```python
from build123d import *
from OCP.BRepFilletAPI import BRepFilletAPI_MakeChamfer

# Parameters (mm, degrees)
SKETCH1_W                      = 70
SKETCH1_H                      = 70
BOSS_EXTRUDE1_DEPTH            = 10
M3_CLEARANCE_HOLE1_D           = 3.4
M3_CLEARANCE_HOLE1_CSINK_D     = 3.65
M3_CLEARANCE_HOLE1_CSINK_ANGLE = 90
SKETCH14_W                     = 70
SKETCH14_H                     = 10
BOSS_EXTRUDE2_DEPTH            = 63
SKETCH13_W                     = 186
SKETCH13_H                     = 106
BOSS_EXTRUDE3_DEPTH            = 10
CHAMFER1_SIZE                  = 40
CHAMFER1_SIZE2                 = 53
HOLE1_D                        = 4.5
HOLE1_DEPTH                    = 9
HOLE1_CBORE_D                  = 5.2
HOLE1_CBORE_DEPTH              = 2
CHAMFER2_SIZE                  = 2
CHAMFER2_SIZE_2                = 0.35


with BuildPart() as part:
    # Sketch1 → Boss-Extrude1 (new body)
    with BuildSketch(Plane.XY):
        Rectangle(SKETCH1_W, SKETCH1_H)
    extrude(amount=BOSS_EXTRUDE1_DEPTH)

    # M3 Clearance Hole1 (through all)
    with Locations(Plane.XY.offset(10)):
        with Locations((6.314276634, -15.244012286), (10.044563579, 13.090330115), (-16.358840213, 2.153682172)):
            CounterSinkHole(M3_CLEARANCE_HOLE1_D / 2, M3_CLEARANCE_HOLE1_CSINK_D / 2, counter_sink_angle=M3_CLEARANCE_HOLE1_CSINK_ANGLE)

    # Sketch14 → Boss-Extrude2 (add)
    with BuildSketch(Plane.XZ.offset(35)):
        with Locations((0, 5)):
            Rectangle(SKETCH14_W, SKETCH14_H)
    extrude(amount=BOSS_EXTRUDE2_DEPTH)

    # Sketch13 → Boss-Extrude3 (add)
    with BuildSketch(Plane.XZ.offset(98)):
        with Locations((0, -43)):
            Rectangle(SKETCH13_W, SKETCH13_H)
    extrude(amount=-BOSS_EXTRUDE3_DEPTH)

    # Chamfer1
    chamfer1_edges = [part.edges().sort_by_distance(p)[0] for p in [
        (0, -88, 0),
    ]]
    chamfer1_side = [part.faces().sort_by_distance(p)[0] for p in [
        (0, -88, -44.766933109),
    ]]
    chamfer(chamfer1_edges, length=CHAMFER1_SIZE, length2=CHAMFER1_SIZE2, reference=chamfer1_side[0])

    # Hole1
    with Locations(Plane(origin=(0, -88, 0), x_dir=(1, 0, 0), z_dir=(0, 1, 0))):
        with Locations((-89, 7.3), (-89, 82.2), (-40.8, 6), (-73.8, 58.1), (-45.9, 58.1)):
            CounterBoreHole(HOLE1_D / 2, HOLE1_CBORE_D / 2, HOLE1_CBORE_DEPTH, depth=HOLE1_DEPTH)

    # Chamfer2
    chamfer2_edges_1 = [part.edges().sort_by_distance(p)[0] for p in [
        (-43.4, -90, -6),
    ]]
    chamfer2_side_1 = [part.faces().sort_by_distance(p)[0] for p in [
        (-43.4, -89.993, -6),
    ]]
    chamfer2_edges_2 = [part.edges().sort_by_distance(p)[0] for p in [
        (-91.6, -90, -82.2),
    ]]
    chamfer2_side_2 = [part.faces().sort_by_distance(p)[0] for p in [
        (-91.6, -89.993, -82.2),
    ]]
    chamfer2_edges_3 = [part.edges().sort_by_distance(p)[0] for p in [
        (-91.6, -90, -7.3),
    ]]
    chamfer2_side_3 = [part.faces().sort_by_distance(p)[0] for p in [
        (-91.6, -89.993, -7.3),
    ]]
    chamfer2_edges_4 = [part.edges().sort_by_distance(p)[0] for p in [
        (-48.5, -90, -58.1),
    ]]
    chamfer2_side_4 = [part.faces().sort_by_distance(p)[0] for p in [
        (-48.5, -89.993, -58.1),
    ]]
    chamfer2_edges_5 = [part.edges().sort_by_distance(p)[0] for p in [
        (-76.4, -90, -58.1),
    ]]
    chamfer2_side_5 = [part.faces().sort_by_distance(p)[0] for p in [
        (-76.4, -89.993, -58.1),
    ]]
    chamfer2 = BRepFilletAPI_MakeChamfer(part.part.solid().wrapped)
    for e in chamfer2_edges_1:
        chamfer2.Add(CHAMFER2_SIZE - 0.0001, CHAMFER2_SIZE_2 - 0.0001, e.wrapped, chamfer2_side_1[0].wrapped)
    for e in chamfer2_edges_2:
        chamfer2.Add(CHAMFER2_SIZE - 0.0001, CHAMFER2_SIZE_2 - 0.0001, e.wrapped, chamfer2_side_2[0].wrapped)
    for e in chamfer2_edges_3:
        chamfer2.Add(CHAMFER2_SIZE - 0.0001, CHAMFER2_SIZE_2 - 0.0001, e.wrapped, chamfer2_side_3[0].wrapped)
    for e in chamfer2_edges_4:
        chamfer2.Add(CHAMFER2_SIZE - 0.0001, CHAMFER2_SIZE_2 - 0.0001, e.wrapped, chamfer2_side_4[0].wrapped)
    for e in chamfer2_edges_5:
        chamfer2.Add(CHAMFER2_SIZE - 0.0001, CHAMFER2_SIZE_2 - 0.0001, e.wrapped, chamfer2_side_5[0].wrapped)
    add(Compound.cast(chamfer2.Shape()), mode=Mode.REPLACE)  # a hair under: the kernel refuses the full size


solid = part.part
```
Part model, mm, in its own coordinate system. A direction names the side the tool comes from. Coordinates: 2 decimals unless noted, no trailing zeros. Write each loop counter-clockwise with the first axis right and the second up, starting at its lowest first coordinate (ties: lowest second). Pieces come first, ordered by that corner, then holes.
Item 1: Mould opens along Z. For faces 4 (the face through (0, 0, 0)), 5 (the face through (-89, -97, -82)), 6 (the face through (93, -93, -44)) say: released by +Z, released by -Z, zero draft, split by the parting line, or undercut.
Item 2: Slice it at C-C (y = -5). Write the cut outline in (x, z).
Item 3: Probe line 1 (X direction, y = -95.5, z = -58.1); line 2 (X direction, y = -93.25, z = -6); line 3 (X direction, y = -81, z = -14). List the from-to ranges inside material, lowest first.
Item 4: Slice it at A-A (x = -4.5). Write the cut outline in (y, z).
Item 5: Which spindle directions (+Z, -Z, +X, -X, +Y, -Y) get a long thin tool onto all of the face, cutting with end or side? Do faces 1 (the face through (-1, -47, 10)), 2 (the face through (-46, -97, -58)), 3 (the face through (-35, -39, 1)). Say none if no direction does.
Item 6: Pin check, flat tips, straight feed: pin 1 (3 mm diameter, centred on x = -16.36, y = 2.15, fed in from +Z); pin 2 (1.4 mm diameter, centred on x = -46, z = -59, fed in from +Y); pin 3 (3 mm diameter, centred on x = -25.5, z = -82.5, fed in from +Y). Stop position of each tip, or through.
Results found:
1. face 4: released by -Z
1. face 5: undercut
1. face 6: zero draft
2. outline: (-35, 0) - (35, 0) - (35, 10) - (-35, 10) - close
3. line 1: x = -93 to -76.05, -71.55 to -48.15, -43.65 to 93
3. line 2: x = -93 to -90.84, -87.16 to -43.05, -38.55 to 93
3. line 3: x = -35 to 35
4. outline: (-98, -96) - (-88, -96) - (-88, -40) - (-35, 0) - (35, 0) - (35, 10) - (-98, 10) - close
5. face 1: +Z, +X, -X, +Y, -Y
5. face 2: +Y
5. face 3: +Z, -Z, -X, +Y
6. pin 1: passes through
6. pin 2: stops at y = -97
6. pin 3: stops at y = -88
